Source: CAD feature listing. Evaluate the final solid. Frame: model axes, mm. A direction names the side the tool comes from. Give positions to 0.01 mm unless a question says otherwise; leave off trailing zeros. Order: outer loops, then holes, each group sorted by start corner. A loop starts at its lowest first (then second) coordinate and runs counter-clockwise, first axis right, second up. Notation, with made-up numbers: (55, -36) -> (73, -36) arc R32 cw to (73, -3) -> close; hole circle Ø8 at (-37.75, 88.25). An arc over 180 degrees is marked (long way). Use CSV: the item, a comma, the result in double quotes.
Autodesk Fusion 360 part; units mm, degrees
sketch "Sketch1" plane through (0, 0, 0) normal (0, 0, 1) x (1, 0, 0)
  line L0 (0, 0) -> (62, 0)
  line L1 (62, 0) -> (62, 13)
  line L2 (62, 13) -> (0, 13)
  line L3 (0, 13) -> (0, 0)
  dimension "d1" = 62
  dimension "d2" = 13
extrude "Extrude1" add sketch "Sketch1" along normal blind 3.5
sketch "Sketch2" plane through (0, 0, 3.5) normal (0, 0, 1) x (-1, 0, 0)
  line L0 (0, -13) -> (0, 0)
  line L1 (0, 0) -> (-62, 0)
  line L2 (-62, 0) -> (-62, -13)
  line L3 (-62, -13) -> (0, -13)
  line L4 (-2.25, 0) -> (-59.75, 0)
  line L5 (-59.75, 0) -> (-59.75, -11)
  line L6 (-59.75, -11) -> (-2.25, -11)
  line L7 (-2.25, -11) -> (-2.25, 0)
  line L8 (-30.25, 0) -> (-59.75, 0)
  line L9 (-59.75, 0) -> (-59.75, -11)
  line L10 (-59.75, -11) -> (-30.25, -11)
  line L11 (-30.25, -11) -> (-30.25, 0)
  dimension "d5" = 57.5
  dimension "d6" = 11
  dimension "d7" = 2.25
  dimension "d8" = 29.5
  dimension "d9" = 11
  dimension "d22" = 2.25
extrude "Extrude7" add sketch "Sketch2" along normal blind 5 contours L1 L4 L6 L7 L11 | L1 L4 L5 L6 L8 L9 L10 L11
sketch "Sketch6" plane through (0, 0, 8.5) normal (0, 0, 1) x (-1, 0, 0)
  line L0 (-2.25, -11) -> (-2.25, 0)
  line L1 (-2.25, 0) -> (-59.75, 0)
  line L2 (-59.75, 0) -> (-59.75, -11)
  line L3 (-59.75, -11) -> (-2.25, -11)
  line L4 (-20, -11) -> (-47.25, -11)
  line L5 (-47.25, -11) -> (-47.25, 0)
  line L6 (-47.25, 0) -> (-20, 0)
  line L7 (-20, 0) -> (-20, -11)
  line L8 (-2.25, -11) -> (-2.25, 0)
  dimension "d30" = 17.75
  dimension "d31" = 27.25
extrude "Extrude9" cut sketch "Sketch6" against normal blind 5 contours L1 L3 L4 L5 L6 L7
fillet "Fillet2" radius 0.5 4 edges at (59.75, 11, 6) (47.25, 11, 6) (20, 11, 6) (2.25, 11, 6)
1. Pin query (flat end, axial travel): P1, Ø4, axis at y = 3, z = 7, coming from the -X side; P2, Ø1.5, axis at y = 3, z = 5, coming from the +X side; P3, Ø6.5, axis at x = 33.5, y = 7, coming from the +Z side. Return the tip coordinate at first contact, or that it passes through.
Answer below:
P1,"stops at x = 2.25"
P2,"stops at x = 59.75"
P3,"stops at z = 3.5"
2. Ray query, line 1 along X through (y, z) = (9.5, 4.75); line 2 along Z through (x, y) = (24, 10.75); line 3 along Y through (x, z) = (14.5, 6.25). Return the intervals inside material, ascending.
Answer below:
line 1,"x = 2.25 to 20, 47.25 to 59.75"
line 2,"z = 0 to 3.5"
line 3,"y = 0 to 11"
3. Mould query, pull axis X, two halves, no side actions, for faces 5 (the flat face through (20, 5, 6)), 6 (the flat face through (62, 6, 2)), 7 (the flat face through (11, 11, 6)), 8 (the flat face through (47.25, 5, 6)). Classes: released by +X, released by -X, zero draft, split by the parting line, or undercut.
Answer below:
face 5,"undercut"
face 6,"released by +X"
face 7,"zero draft"
face 8,"undercut"
4. Section query A-A on z = 5.5. Return loops of the section in (x, y).
Answer below:
outline,"(2.25, 0) -> (20, 0) -> (20, 10.5) arc R0.5 ccw to (19.5, 11) -> (2.75, 11) arc R0.5 ccw to (2.25, 10.5) -> close; (47.25, 0) -> (59.75, 0) -> (59.75, 10.5) arc R0.5 ccw to (59.25, 11) -> (47.75, 11) arc R0.5 ccw to (47.25, 10.5) -> close"
5. Section query B-B on x = 11. Return loops of the section in (y, z), plus the area to 4 significant figures.
Answer below:
outline,"(0, 0) -> (13, 0) -> (13, 3.5) -> (11, 3.5) -> (11, 8.5) -> (0, 8.5) -> close"
area,"100.5 mm²"
6. Section query D-D on x = 39.5. Return loops of the section in (y, z), plus the area to 3 significant figures.
Answer below:
outline,"(0, 0) -> (13, 0) -> (13, 3.5) -> (0, 3.5) -> close"
area,"45.5 mm²"
7. Access query for faces 1 (the flat face through (31, 7, 3.5)), 2 (the flat face through (2.25, 5, 6)), 3 (the flat face through (54, 11, 6)), 4 (the flat face through (59.75, 5, 6)). Directions: +Z, -Z, +X, -X, +Y, -Y. A direction counts if a zero-diameter tool reaches every point of the face in a straight line with its end or side. Return the directions, or none.
Answer below:
face 1,"+Z, +Y"
face 2,"+Z, -X, +Y, -Y"
face 3,"+Z, +X, -X, +Y"
face 4,"+Z, +X, +Y, -Y"
8. Section query C-C on y = 3.5. Return loops of the section in (x, z), plus the area to 3 significant figures.
Answer below:
outline,"(0, 0) -> (62, 0) -> (62, 3.5) -> (59.75, 3.5) -> (59.75, 8.5) -> (47.25, 8.5) -> (47.25, 3.5) -> (20, 3.5) -> (20, 8.5) -> (2.25, 8.5) -> (2.25, 3.5) -> (0, 3.5) -> close"
area,"368 mm²"
